For this review, take the finished solid that the model builds, in its own axes (mm). Face numbers are marked on the shaded views. A direction names the side the tool comes from. Round coordinates to 2 decimals unless told otherwise and drop trailing zeros. Write each loop counter-clockwise with the first axis right and the second up, starting at its lowest first coordinate (ties: lowest second). Pieces come first, ordered by that corner, then holes. Notation, with made-up numbers: (21, -19) - (35, -19) arc R14 ccw to (35, 1) - close; hole circle Ø2 at (4, 32.5). An arc over 180 degrees is marked (long way). Answer in a Markdown table with one row per item. Add a question column.
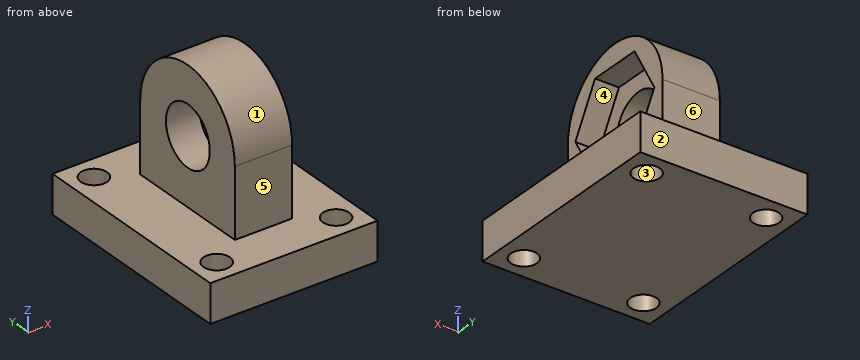
from build123d import *

# Parameters (mm, degrees)
SKETCH001_W            = 17.5
SKETCH001_H            = 22.5
SKETCH001_R            = 2.75
PAD_DEPTH              = 8
SKETCH001_MIRRORED_2_W = 17.5
SKETCH001_MIRRORED_2_H = 22.5
SKETCH001_MIRRORED_2_R = 2.75
PAD_MIRRORED_2_DEPTH   = 8
SKETCH003_W            = 12
SKETCH003_H            = 27
PAD001_DEPTH           = 28
POCKET_DEPTH           = 56
SKETCH006_R            = 6.25
POCKET001_DEPTH        = 23.820636
POCKET001_DEPTH_BACK   = -11.181364
POCKET002_DEPTH        = 5


with BuildPart() as part:
    # Sketch001 → Pad (new body)
    with BuildSketch(Plane.XY):
        with Locations((8.75, 11.25)):
            Rectangle(SKETCH001_W, SKETCH001_H)
        with Locations((12.5, 17.5)):
            Circle(SKETCH001_R, mode=Mode.SUBTRACT)
    pad = extrude(amount=PAD_DEPTH)

    # Sketch001 Mirrored 2 → Pad Mirrored 2 (add)
    with BuildSketch(Plane(origin=(0, 0, 0), x_dir=(-1, 0, 0), z_dir=(0, 0, -1))):
        with Locations((8.75, 11.25)):
            Rectangle(SKETCH001_MIRRORED_2_W, SKETCH001_MIRRORED_2_H)
        with Locations((12.5, 17.5)):
            Circle(SKETCH001_MIRRORED_2_R, mode=Mode.SUBTRACT)
    pad_mirrored_2 = extrude(amount=-PAD_MIRRORED_2_DEPTH)

    # Mirrored001: Pad, Pad Mirrored 2 across Sketch001 H_Axis
    add(pad.mirror(Plane.ZX))
    add(pad_mirrored_2.mirror(Plane.ZX))

    # Sketch003 (on Face12 of MultiTransform) → Pad001 (join)
    with BuildSketch(Plane.XY.offset(8)):
        with Locations((0.319636, 0.107343)):
            Rectangle(SKETCH003_W, SKETCH003_H)
    extrude(amount=PAD001_DEPTH)

    # Sketch004 (on Face23 of Pad001) → Pocket (cut)
    with BuildSketch(Plane(origin=(-5.680364, 0, 0), x_dir=(0, -1, 0), z_dir=(-1, 0, 0))):
        with BuildLine():
            ThreePointArc((13.392657, 22.424454), (-0.107343, 35.924454), (-13.607343, 22.424454))
            Line((-13.607343, 22.424454), (-13.627651, 49.129635))
            Line((-13.627651, 49.129635), (14.64682, 49.129635))
            Line((14.64682, 49.129635), (13.392657, 22.424454))
        make_face()
    extrude(amount=-POCKET_DEPTH, mode=Mode.SUBTRACT)

    # Sketch006 (on Face12 of Pocket) → Pocket001 (cut, two sides)
    with BuildSketch(Plane.YZ.offset(6.319636)) as pocket001_sk:
        with Locations((0, 22)):
            Circle(SKETCH006_R)
    extrude(amount=-POCKET001_DEPTH, mode=Mode.SUBTRACT)
    extrude(pocket001_sk.sketch, amount=-POCKET001_DEPTH_BACK, mode=Mode.SUBTRACT)

    # Sketch007 (on Face12 of Pocket001) → Pocket002 (cut)
    with BuildSketch(Plane.YZ.offset(6.319636)):
        Polygon((5.629165, 12.25), (11.25833, 22), (5.629165, 31.75), (-5.629165, 31.75), (-11.25833, 22), (-5.629165, 12.25), align=None)
    extrude(amount=-POCKET002_DEPTH, mode=Mode.SUBTRACT)


solid = part.part
Q1. To check wall thickness, follow probe 1 along Y at (x, z) = (-12.5, 2.5); probe 2 along X at (y, z) = (-17.5, 3.75); probe 3 along Z at (x, y) = (11.5, 7.5). State the ranges of each line that lie inside material, in increasing order.
Q2. Add section A-A on x = -12.5. State the section outline as (y, z) points.
Q3. Add section B-B on y = 17.5. State the section outline as (x, z) points.
Q4. Tool access review of the marked faces 4, 5 and 6: name each direction out of +Z, -Z, +X, -X, +Y, -Y from which nothing blocks a thin tool from reaching the whole face with its end or side.
Q5. Add section D-D on z = 6. State the section outline as (x, y) points.
Q6. Draft analysis for pull direction Y (two halves, no side actions). For the marked faces 1, 2 and 3, state which applies: released by +Y, released by -Y, zero draft, split by the parting line, or undercut.
Q7. Insertion check: pin 1 Ø2 at (x, y) = (-0.5, -15) entering from +Z; pin 2 Ø1.5 at (x, y) = (3, -2) entering from +Z; pin 3 Ø20 at (y, z) = (0, 22) entering from +X. Each pin has a flat end and moves straight along its axis. Give the tip position at first contact, or say it passes through.
Q8. Add section C-C on z = 27. State the section outline as (x, y) points.
Answer sheet:
| question | item | result |
|---|---|---|
| 1 | probe 1 | y = -22.5 to -20.25, -14.75 to 14.75, 20.25 to 22.5 |
| 1 | probe 2 | x = -17.5 to -15.25, -9.75 to 9.75, 15.25 to 17.5 |
| 1 | probe 3 | z = 0 to 8 |
| 2 | outline | (-22.5, 0) - (-20.25, 0) - (-20.25, 8) - (-22.5, 8) - close; (-14.75, 0) - (14.75, 0) - (14.75, 8) - (-14.75, 8) - close; (20.25, 0) - (22.5, 0) - (22.5, 8) - (20.25, 8) - close |
| 3 | outline | (-17.5, 0) - (-15.25, 0) - (-15.25, 8) - (-17.5, 8) - close; (-9.75, 0) - (9.75, 0) - (9.75, 8) - (-9.75, 8) - close; (15.25, 0) - (17.5, 0) - (17.5, 8) - (15.25, 8) - close |
| 4 | face 4 | +X |
| 4 | face 5 | +Z, +X, -X, -Y |
| 4 | face 6 | +Z, +X, -X, +Y |
| 5 | outline | (-17.5, -22.5) - (17.5, -22.5) - (17.5, 22.5) - (-17.5, 22.5) - close; hole circle Ø5.5 at (-12.5, -17.5); hole circle Ø5.5 at (-12.5, 17.5); hole circle Ø5.5 at (12.5, -17.5); hole circle Ø5.5 at (12.5, 17.5) |
| 6 | face 1 | split by the parting line |
| 6 | face 2 | released by +Y |
| 6 | face 3 | undercut |
| 7 | pin 1 | stops at z = 8 |
| 7 | pin 2 | stops at z = 35.86 |
| 7 | pin 3 | stops at x = 6.32 |
| 8 | outline | (-5.68, -12.59) - (6.32, -12.59) - (6.32, -8.37) - (1.32, -8.37) - (1.32, -3.75) - (-5.68, -3.75) - close; (-5.68, 3.75) - (1.32, 3.75) - (1.32, 8.37) - (6.32, 8.37) - (6.32, 12.81) - (-5.68, 12.81) - close |
